The model under review builds one solid part; all positions refer to its coordinate system, in mm. A direction names the side the tool comes from. Give positions to 0.01 mm unless a question says otherwise; leave off trailing zeros. Order: outer loops, then holes, each group sorted by start corner. A loop starts at its lowest first (then second) coordinate and runs counter-clockwise, first axis right, second up. Notation, with made-up numbers: (26.5, 41) - (77.5, 41) arc R14 ccw to (77.5, 63) - close; hole circle Ø8 at (8.25, -6.5). An arc over 180 degrees is marked (long way). Use CSV: the item, a comma, the result in double quotes. Start each with the question number.
```python
from build123d import *


with BuildPart() as part:
    # Esquisse1 → Révolution1 (revolve)
    with BuildSketch(Plane.XY, mode=Mode.PRIVATE) as r_volution1_sk:
        with BuildLine():
            Line((0, 70), (0, 10))
            Line((0, 10), (448, 10))
            Line((448, 10), (448, 70))
            Line((448, 70), (320.5, 70))
            ThreePointArc((320.5, 70), (314.136038969, 67.363961031), (311.5, 61))
            Line((311.5, 61), (311.5, 60))
            Line((311.5, 60), (136.5, 60))
            Line((136.5, 60), (136.5, 61))
            ThreePointArc((136.5, 61), (133.863961031, 67.363961031), (127.5, 70))
            Line((127.5, 70), (0, 70))
        make_face()
    revolve(r_volution1_sk.sketch.rotate(Axis((0, 0, 0), (1, 0, 0)), 90), axis=Axis((0, 0, 0), (1, 0, 0)))


solid = part.part
```
1. Consider section C-C (x = 50.5). Give the boundary of the cut face in (y, z), and give its area (3 significant figures).
2. Mouldability with a two-part tool opening along X and no side actions: class faces 1 (the face through (448, 15, 1)), 2 (the face through (383.358, 68.335, -15.175)), 3 (the face through (222.78, -50.59, 32.26)), 4 (the face through (311.5, 40, 45)) as pulls with the +X half, pulls with the -X half, needs draft (parallel to the pull), parting line crosses it, or undercut.
3. Consider section D-D (x = 150). Give the boundary of the cut face in (y, z).
4. To check wall thickness, follow L1, parallel to Y at x = 171, z = 0; L2, parallel to Y at x = 320, z = 0; L3, parallel to X at y = 63.5, z = -21.5. State the ranges of each line that lie inside material, in increasing order. Write a range as [from, to].
5. Clearance check with flat-ended pins moving along their axes: pin 1 (3 mm diameter, centred on x = 77.5, z = 33, fed in from +Y); pin 2 (6 mm diameter, centred on x = 170.5, y = 48, fed in from -Z); pin 3 (2 mm diameter, centred on x = 181.5, y = 1, fed in from +Z). State where each tip first meets the part, or that it passes through.
6. Tool access review of faces 5 (the face through (0, 15, -1)), 6 (the face through (136.5, 40, -45)): name each direction out of +Z, -Z, +X, -X, +Y, -Y from which nothing blocks a thin tool from reaching the whole face with its end or side.
7. Consider section A-A (y = 0). Give the boundary of the cut face in (x, z).
Answers follow:
1,outline,"circle Ø140 at (0, 0); hole circle Ø20 at (0, 0)"
1,area,"15,100 mm^2"
2,face 1,"pulls with the +X half"
2,face 2,"needs draft"
2,face 3,"undercut"
2,face 4,"undercut"
3,outline,"circle Ø120 at (0, 0); hole circle Ø20 at (0, 0)"
4,L1,"y = [-60, -10], [10, 60]"
4,L2,"y = [-69.99, -10], [10, 69.99]"
4,L3,"x = [0, 134.17], [313.83, 448]"
5,pin 1,"stops at y = 62.51"
5,pin 2,"stops at z = -39.69"
5,pin 3,"stops at z = 60"
6,face 5,"+Z, -Z, -X, +Y, -Y"
6,face 6,"none"
7,outline,"(0, -70) - (127.5, -70) arc R9 ccw to (136.5, -61) - (136.5, -60) - (311.5, -60) - (311.5, -61) arc R9 ccw to (320.5, -70) - (448, -70) - (448, -10) - (0, -10) - close; (0, 10) - (448, 10) - (448, 70) - (320.5, 70) arc R9 ccw to (311.5, 61) - (311.5, 60) - (136.5, 60) - (136.5, 61) arc R9 ccw to (127.5, 70) - (0, 70) - close"
